Could you check a few things on this drawing? It's one solid part, dimensions in mm from its lowest x, y, z. Coordinates: 2 decimals unless noted, no trailing zeros. Write each loop counter-clockwise with the first axis right and the second up, starting at its lowest first coordinate (ties: lowest second). Pieces come first, ordered by that corner, then holes. Notation, with made-up numbers: (85, -19) - (141, -19) arc R30 cw to (141, 13) - close; hole circle Ø4 at (44.25, 80). An arc over 180 degrees is marked (long way). Write item = value, one per line. Start each with the question number.
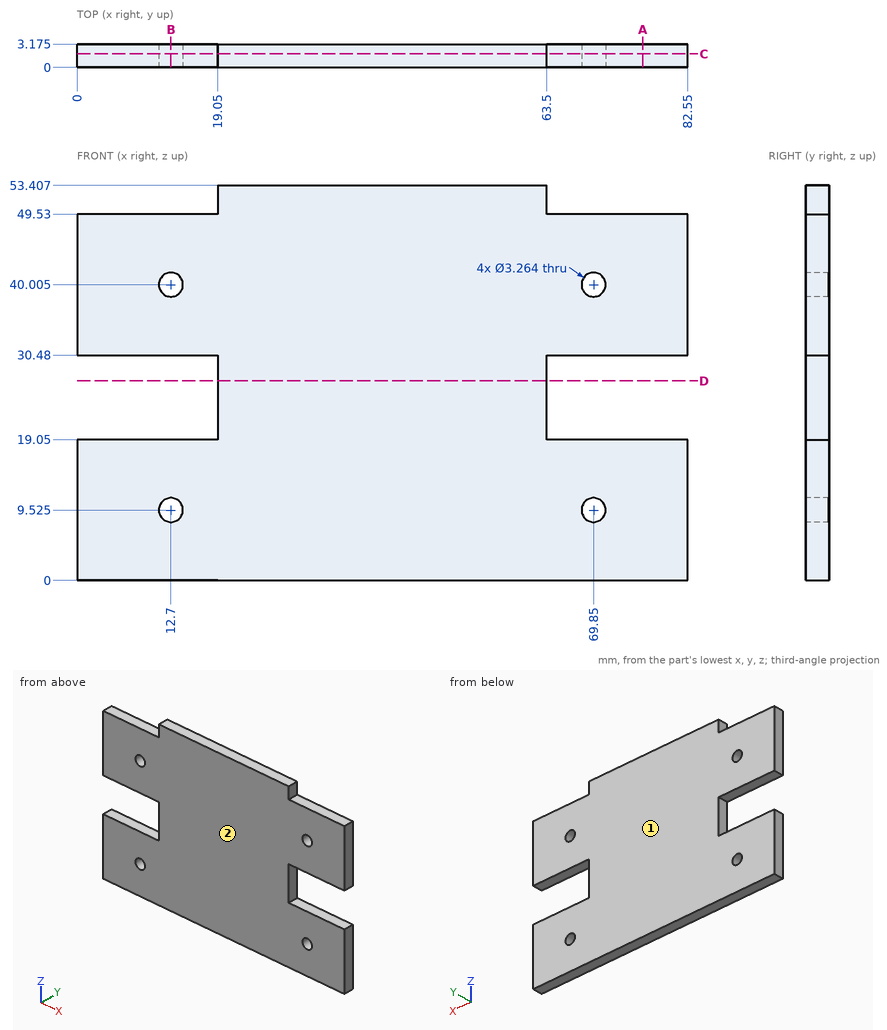
1) Suppose I cut it at B-B on x = 12.7. Please give me the cut outline in (y, z) (3 decimals), plus the area to 3 significant figures.
2) If I drill on probe 1 along Z at (x, y) = (12.7, 1.6); probe 2 along Z at (x, y) = (76, 2.4); probe 3 along X at (y, z) = (1.1, 39.5), over which ranges is the centre line in solid material (lowest first)? Write a range as [from, to].
3) Suppose I cut it at A-A on x = 76.5. Please give me the cut outline in (y, z) (3 decimals).
4) Thinking about a two-plate mould opening in Y: for the marked faces 1 and 2, which applies, +Y half, -Y half, draft (parallel to the pull), parting line (faces both ways), or undercut?
5) Suppose I cut it at D-D on z = 27. Please give me the cut outline in (x, y) (3 decimals), plus the area to 3 significant figures.
6) For P1, Ø1.6, axis at y = 2.5, z = 52, coming from the -X side; P2, Ø1.6, axis at x = 5.5, y = 2.5, coming from the +Z side; P3, Ø4, axis at x = 69.85, z = 9.525, coming from the +Y side (3 decimals), each with a flat end and sliding along its axis, tell me the tip position at first contact or that it passes through.
7) Suppose I cut it at C-C on y = 1.85. State how many separate pieces and enclosed holes the cut face has, plus the area to 3 significant figures.
Reply:
q1.outline = (0, 0) - (3.175, 0) - (3.175, 7.893) - (0, 7.893) - close; (0, 11.157) - (3.175, 11.157) - (3.175, 19.05) - (0, 19.05) - close; (0, 30.48) - (3.175, 30.48) - (3.175, 38.373) - (0, 38.373) - close; (0, 41.637) - (3.175, 41.637) - (3.175, 49.53) - (0, 49.53) - close
q1.area = 100 mm^2
q2.probe_1 = [0, 7.89], [11.16, 19.05], [30.48, 38.37], [41.64, 49.53]
q2.probe_2 = [0, 19.05], [30.48, 49.53]
q2.probe_3 = [0, 11.15], [14.25, 68.3], [71.4, 82.55]
q3.outline = (0, 0) - (3.175, 0) - (3.175, 19.05) - (0, 19.05) - close; (0, 30.48) - (3.175, 30.48) - (3.175, 49.53) - (0, 49.53) - close
q4.face_1 = +Y half
q4.face_2 = -Y half
q5.outline = (19.05, 0) - (63.5, 0) - (63.5, 3.175) - (19.05, 3.175) - close
q5.area = 141 mm^2
q6.P1 = 19.05
q6.P2 = 49.53
q6.P3 = 3.175
q7.separate_pieces = 1
q7.enclosed_holes = 4
q7.area = 3,790 mm^2
